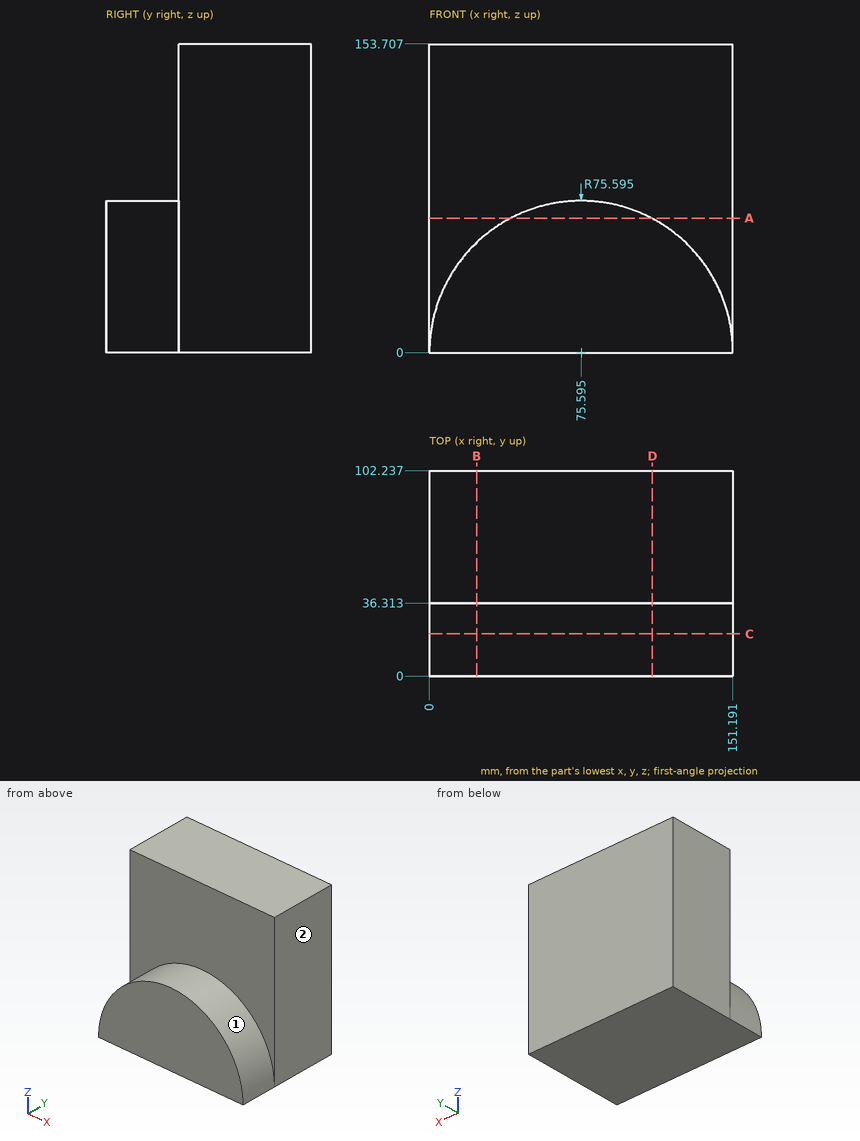
Geometry check sheet. Reference: drawing and pictorial views, mm from the part's lowest x, y, z. A direction names the side the tool comes from. Give positions to 0.01 mm unless a question says otherwise; leave off trailing zeros. Loops run counter-clockwise (first coordinate to the right, second up) from the corner with the lowest first, then second, coordinate; pieces in that order, holes last.
1. Thickness scan on line 1 (Y direction, x = 92, z = 130); line 2 (Z direction, x = 29.5, y = 35.5) (1 decimal); line 3 (Z direction, x = 119.5, y = 10.5). Record the ranges inside material, lowest first.
2. Section check C-C, the plane y = 21. Enter the section's corners in (x, z) (1 decimal).
3. Set-up check for the marked faces 1 and 2: record each of +Z, -Z, +X, -X, +Y, -Y from which the full face is reachable in a straight line by a thin tool's end or side.
4. Section check A-A, the plane z = 67. Enter the section's corners in (x, y) (1 decimal).
5. Section check B-B, the plane x = 23.5. Enter the section's corners in (y, z).
6. Go/stop test with flat-tipped pins: pin 1 Ø12 at (y, z) = (29.5, 19) entering from -X; pin 2 Ø12 at (y, z) = (17, 68) entering from +X (1 decimal). Record where each tip stops, or that it passes through.
7. Section check D-D, the plane x = 111. Enter the section's corners in (y, z), then the cut area to 3 significant figures.
Geometry says:
1. line 1: y = 36.31 to 102.24
1. line 2: z = 0 to 59.9
1. line 3: z = 0 to 61.54
2. outline: (0, 0) - (151.2, 0) arc R75.6 ccw to start
3. face 1: +Z, -Y
3. face 2: +Z, -Z, +X, +Y, -Y
4. outline: (0, 36.3) - (40.6, 36.3) - (40.6, 0) - (110.6, 0) - (110.6, 36.3) - (151.2, 36.3) - (151.2, 102.2) - (0, 102.2) - close
5. outline: (0, 0) - (102.24, 0) - (102.24, 153.71) - (36.31, 153.71) - (36.31, 54.78) - (0, 54.78) - close
6. pin 1: stops at x = 1.13
6. pin 2: stops at x = 118.8
7. outline: (0, 0) - (102.24, 0) - (102.24, 153.71) - (36.31, 153.71) - (36.31, 66.79) - (0, 66.79) - close
7. area: 12,600 mm2
